from build123d import *

# Parameters (mm, degrees)
F0_W     = 306.4280003309
F0_H     = 170.664742589
F0_W_2   = 291.2639975548
F0_H_2   = 149.4066938758
F1_DEPTH = 101.6
F2_W     = 138.0773968995
F2_H     = 67.8825782061
F3_DEPTH = 25.4
F4_DEPTH = 219.202
F5_R     = 19.4558294746
F6_DEPTH = 25.4
F7_DEPTH = 393.7


with BuildPart() as f1:
    # F0 (on Top) → F1 (new body)
    with BuildSketch(Plane.XY):
        with Locations((-1.1102333665, -0.0495761633)):
            Rectangle(F0_W, F0_H)
        with Locations((-3.4452080727, 0.6861723959)):
            Rectangle(F0_W_2, F0_H_2, mode=Mode.SUBTRACT)
    extrude(amount=F1_DEPTH)

    # F2 (on face) → F3 (join)
    with BuildSketch(Plane.XZ.offset(85.3819474578)):
        with Locations((9.856319055, 84.741289103)):
            Rectangle(F2_W, F2_H)
    extrude(amount=F3_DEPTH)

    # F4 (cut): a face of the model
    f4_faces = [f1.faces().sort_by_distance(p)[0] for p in [
        (9.856319055, -110.7819474578, 84.741289103),
    ]]
    extrude(f4_faces, amount=-F4_DEPTH, mode=Mode.SUBTRACT)

    # F5 (on face) → F6 (join)
    with BuildSketch(Plane(origin=(-154.324233532, 0, 0), x_dir=(0, -1, 0), z_dir=(-1, 0, 0))):
        with Locations((0, 55.4958842695)):
            Circle(F5_R)
    extrude(amount=F6_DEPTH)

    # F7 (cut): a face of the model
    f7_faces = [f1.faces().sort_by_distance(p)[0] for p in [
        (-179.724233532, 0, 55.4958842695),
    ]]
    extrude(f7_faces, amount=-F7_DEPTH, mode=Mode.SUBTRACT)


solid = f1.part
Can you work these out from the model? Positions are in its coordinate system, mm. A direction names the side the tool comes from. Give positions to 0.01 mm unless a question says otherwise; leave off trailing zeros. Order: outer loops, then holes, each group sorted by start corner. A loop starts at its lowest first (then second) coordinate and runs counter-clockwise, first axis right, second up. Notation, with made-up numbers: M -3.75,-19.75 L 34.25,-19.75 A26 cw 34.25,4.25 Z; hole C 13.5,35 d7. An arc over 180 degrees is marked long. Use a Markdown table: item, result. Add a question column.
Item 1: We'd pull the mould along X, two halves only. Please class faces 1 (the flat face through (-149.077, 16, 39)), 2 (the flat face through (-3, 85.283, 39)), 3 (the flat face through (-154.324, -20, 50)): +X half, -X half, draft (parallel to the pull), parting line (faces both ways), or undercut.
Item 2: For faces 4 (the flat face through (-149.3, -6, 101.6)), 5 (the flat face through (142.187, 16, 39)), 6 (the flat face through (9, -80, 50.8)), which set-ups out of +Z, -Z, +X, -X, +Y, -Y let a thin tool reach every point of the face, with its end or its side?
Item 3: If I drill on L1, parallel to X at y = 29, z = 88; L2, parallel to Z at x = -152.35, y = 0; L3, parallel to Y at x = 72, z = 15, over which ranges is the centre line in solid material (lowest first)? Write a range as [from, to].
Item 4: Will this pin go through, and if not, where does the flat tip stop? pin 1 (3.5 mm diameter, centred on x = -17, y = -79.5, fed in from +Z).
Item 5: Suppose I cut it at B-B (z = 15). List the corners of the cut face in (x, y) for me.
Item 6: Suppose I cut it at A-A (y = 0). List the corners of the cut face in (x, z) for me.
Item 7: Suppose I cut it at C-C (x = 130.5). List the corners of the cut face in (y, z) for me, then the cut area to 3 significant figures.
Item 8: Suppose I cut it at D-D (z = 87). List the corners of the cut face in (x, y) for me, then the cut area to 3 significant figures.
Answer sheet:
| question | item | result |
|---|---|---|
| 1 | face 1 | undercut |
| 1 | face 2 | draft |
| 1 | face 3 | -X half |
| 2 | face 4 | +Z, +X, -X, +Y, -Y |
| 2 | face 5 | +Z, -Z |
| 2 | face 6 | +Z, +Y, -Y |
| 3 | L1 | x = [-154.32, -149.08], [142.19, 152.1] |
| 3 | L2 | z = [0, 36.04], [74.95, 101.6] |
| 3 | L3 | y = [-85.38, -74.02], [75.39, 85.28] |
| 4 | pin 1 | stops at z = 50.8 |
| 5 | outline | M -154.32,-85.38 L 152.1,-85.38 L 152.1,85.28 L -154.32,85.28 Z; hole M -149.08,-74.02 L 142.19,-74.02 L 142.19,75.39 L -149.08,75.39 Z |
| 6 | outline | M -154.32,0 L -149.08,0 L -149.08,36.04 L -154.32,36.04 Z; M -154.32,74.95 L -149.08,74.95 L -149.08,101.6 L -154.32,101.6 Z; M 142.19,0 L 152.1,0 L 152.1,36.04 L 142.19,36.04 Z; M 142.19,74.95 L 152.1,74.95 L 152.1,101.6 L 142.19,101.6 Z |
| 7 | outline | M -85.38,0 L -74.02,0 L -74.02,101.6 L -85.38,101.6 Z; M 75.39,0 L 85.28,0 L 85.28,101.6 L 75.39,101.6 Z |
| 7 | area | 2,160 mm² |
| 8 | outline | M -154.32,-85.38 L -59.18,-85.38 L -59.18,-74.02 L -149.08,-74.02 L -149.08,75.39 L -59.18,75.39 L -59.18,85.28 L -154.32,85.28 Z; M 78.9,-85.38 L 152.1,-85.38 L 152.1,85.28 L 78.9,85.28 L 78.9,75.39 L 142.19,75.39 L 142.19,-74.02 L 78.9,-74.02 Z |
| 8 | area | 5,840 mm² |
